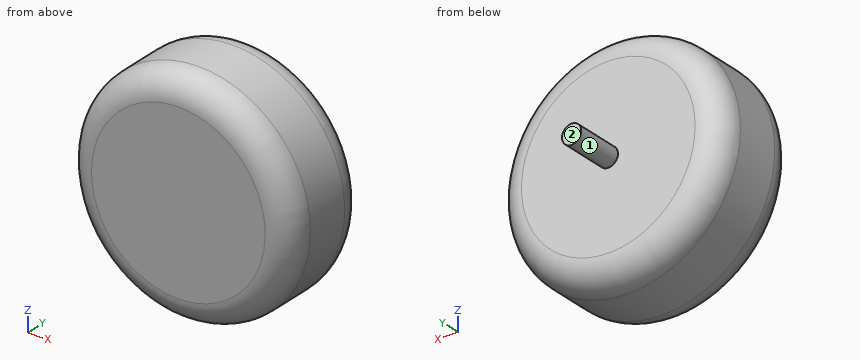
Autodesk Inventor part; units mm, degrees
ref_plane "YZ Plane" through (0, 0, 0) normal (1, 0, 0) x (0, 1, 0)
ref_plane "XZ Plane" through (0, 0, 0) normal (0, 1, 0) x (-1, 0, 0)
ref_plane "XY Plane" through (0, 0, 0) normal (0, 0, 1) x (1, 0, 0)
sketch "Sketch1" plane through (0, 0, 0) normal (0, 1, 0) x (-1, 0, 0)
  circle A0 centre (0, 0) radius 70
  dimension "d4" = 140
extrude "Extrusion1" add sketch "Sketch1" along normal blind 60
sketch "Sketch2" plane through (0, 60, 0) normal (0, 1, 0) x (1, 0, 0)
  circle A0 centre (0, 0) radius 70 construction
  circle A1 centre (0, 0) radius 6
  dimension "d5" = 12
extrude "Extrusion2" add sketch "Sketch2" along normal blind 30
fillet "Fillet1" radius 16 2 edges at (70, 60, 0) (70, 0, 0)
properties part number "GiroMotor"
For this review, take the finished solid that the model builds, in its own axes (mm). Face numbers are marked on the shaded views. A direction names the side the tool comes from. Give positions to 0.01 mm unless a question says otherwise; leave off trailing zeros. Write each loop counter-clockwise with the first axis right and the second up, starting at its lowest first coordinate (ties: lowest second). Pieces come first, ordered by that corner, then holes. Notation, with made-up numbers: M 13,75.25 L 40,75.25 A25 cw 40,100.25 Z; hole C 45.5,34.5 d3. An arc over 180 degrees is marked long. Answer as CSV lines item,"result".
1. For pin 1 (3 mm diameter, centred on x = -22, z = 36, fed in from -Y); pin 2 (8 mm diameter, centred on x = -10.5, z = -23.5, fed in from +Y); pin 3 (1 mm diameter, centred on y = 74.5, z = -1, fed in from -X); pin 4 (3 mm diameter, centred on y = 26, z = 34.5, fed in from +X), all flat-tipped, find the tip position at first contact; note any pin that passes through.
Findings:
pin 1,"stops at y = 0"
pin 2,"stops at y = 60"
pin 3,"stops at x = -5.98"
pin 4,"stops at x = 61.73"
2. Consider section C-C, the plane y = 54. Write out the cut boundary in (x, z), then the cut area to 3 significant figures.
Findings:
outline,"C 0,0 d132.98"
area,"13,900 mm2"
3. Consider section B-B, the plane x = 0. Write out the cut boundary in (y, z), then the cut area to 3 significant figures.
Findings:
outline,"M 0,-54 A16 ccw 16,-70 L 44,-70 A16 ccw 60,-54 L 60,-6 L 90,-6 L 90,6 L 60,6 L 60,54 A16 ccw 44,70 L 16,70 A16 ccw 0,54 Z"
area,"8,540 mm2"
4. For the marked faces 1 and 2, list the 3-axis set-ups (+Z, -Z, +X, -X, +Y, -Y) from which the entire face can be reached by the end or side of a thin tool; tool diameter is ignored.
Findings:
face 1,"+Y"
face 2,"+Z, -Z, +X, -X, +Y"
5. Wall thickness on line 1 (Y direction, x = -4.5, z = 18); line 2 (X direction, y = 5, z = -14.5); line 3 (Y direction, x = 31, z = -49.5): over which ranges is each line inside the solid? List them lowest first.
Findings:
line 1,"y = 0 to 60"
line 2,"x = -64 to 64"
line 3,"y = 0.62 to 59.38"
6. Consider section D-D, the plane y = 38.5. Write out the cut boundary in (x, z).
Findings:
outline,"C 0,0 d140"
7. Consider section A-A, the plane z = 0. Write out the cut boundary in (x, y), then the cut area to 3 significant figures.
Findings:
outline,"M -70,16 A16 ccw -54,0 L 54,0 A16 ccw 70,16 L 70,44 A16 ccw 54,60 L 6,60 L 6,90 L -6,90 L -6,60 L -54,60 A16 ccw -70,44 Z"
area,"8,540 mm2"
